Could you check a few things on this model? Use its own coordinates, in mm. Give positions to 0.01 mm unless a question says otherwise; leave off trailing zeros. Order: outer loops, then holes, each group sorted by start corner. A loop starts at its lowest first (then second) coordinate and runs counter-clockwise, first axis right, second up. Notation, with made-up numbers: (-38.75, 34) -> (6.25, 34) arc R17 cw to (6.25, 51) -> close; hole circle Ø1 at (41.5, 7.5). An arc over 180 degrees is marked (long way). Answer as CSV lines item,"result". Start each with the question number.
(1) I need wall thicknesses on L1, parallel to Z at x = 3.5, y = 0; L2, parallel to Y at x = 6.25, z = -5.25; L3, parallel to Y at x = 1.5, z = 1.75. Which ranges of each line are inside material? Lowest first, please.
(2) We'd pull the mould along Z, two halves only. Please class faces 1 (the face through (3.13, -1.38, 6.2)), 2 (the face through (3.131, 187.577, 0.215)), 3 (the face through (3, 88, 9.779)): released by +Z, released by -Z, zero draft, split by the parting line, or undercut.
(3) I want a section at A-A (z = 0). Please give me the cut outline in (x, y).
Autodesk Inventor part; units mm, degrees
ref_plane "YZ Plane" through (0, 0, 0) normal (1, 0, 0) x (0, 1, 0)
ref_plane "XZ Plane" through (0, 0, 0) normal (0, 1, 0) x (-1, 0, 0)
ref_plane "XY Plane" through (0, 0, 0) normal (0, 0, 1) x (1, 0, 0)
sketch "Sketch1" plane through (0, 0, 0) normal (1, 0, 0) x (0, 1, 0)
  circle A0 centre (0, 0) radius 6.35
  arc A1 (0, 9.779) -> (0, -9.779) centre (0, 0) ccw
  line L0 (0, 9.779) -> (177.8, 9.779)
  line L1 (0, -9.779) -> (177.8, -9.779)
  arc A2 (177.8, -9.779) -> (177.8, 9.779) centre (177.8, 0) ccw
  circle A3 centre (177.8, 0) radius 6.35
  dimension "d0" = 12.7
  dimension "d1" = 19.558
  dimension "d2" = 177.8
  dimension "d3" = 177.8
  dimension "d4" = 12.7
extrude "Extrusion1" add sketch "Sketch1" along normal blind 6.35
properties part number "RollerArm"
Final values:
1,L1,"-9.78 to -6.35, 6.35 to 9.78"
1,L2,"-8.25 to -3.57, 3.57 to 174.23, 181.37 to 186.05"
1,L3,"-9.62 to -6.1, 6.1 to 171.7, 183.9 to 187.42"
2,face 1,"undercut"
2,face 2,"split by the parting line"
2,face 3,"released by +Z"
3,outline,"(0, -9.78) -> (6.35, -9.78) -> (6.35, -6.35) -> (0, -6.35) -> close; (0, 6.35) -> (6.35, 6.35) -> (6.35, 171.45) -> (0, 171.45) -> close; (0, 184.15) -> (6.35, 184.15) -> (6.35, 187.58) -> (0, 187.58) -> close"
